from build123d import *

# Parameters (mm, degrees)
F0_W     = 38.1
F0_H     = 38.1
F1_DEPTH = 25.4
F3_DEPTH = 50.8
F4_DEPTH = 6.35


with BuildPart() as f1:
    # F0 (on Front) → F1 (new body)
    with BuildSketch(Plane.XZ):
        with Locations((19.05, 19.05)):
            Rectangle(F0_W, F0_H)
    extrude(amount=F1_DEPTH)

    # F2 (on face) → F3 (cut)
    with BuildSketch(Plane.YZ.offset(38.1)):
        Polygon((-12.6932453566, 11.4907970736), (-12.6932453566, 38.1), (-25.4, 38.1), (-25.4, 11.4952089814), (-25.3932453566, 11.4907970736), align=None)
    extrude(amount=-F3_DEPTH, mode=Mode.SUBTRACT)

    # F4 (cut): a face of the model
    f4_faces = [f1.faces().sort_by_distance(p)[0] for p in [
        (19.05, -6.3466226783, 38.1),
    ]]
    extrude(f4_faces, amount=-F4_DEPTH, mode=Mode.SUBTRACT)


solid = f1.part
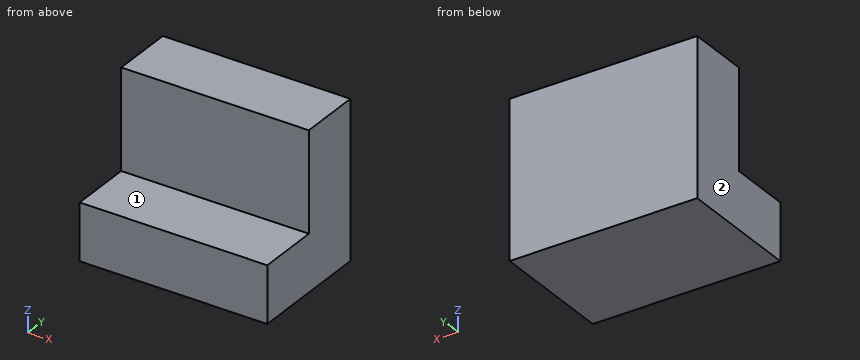
Can you work these out from the model? Positions are in its coordinate system, mm. Face numbers are marked on the shaded views. A direction names the side the tool comes from. Give positions to 0.01 mm unless a question says otherwise; leave off trailing zeros. Loops run counter-clockwise (first coordinate to the right, second up) from the corner with the lowest first, then second, coordinate; pieces in that order, holes last. Notation, with made-up numbers: M 25.25,-37 L 37.25,-37 A15 cw 37.25,-25 Z; hole C 51.25,64.5 d1. An arc over 180 degrees is marked long. One line per item, written item: value. Start each with the question number.
1) If we section it at B-B, the plane z = 12: Write out the boundary of the cut face in (x, y).
2) On a 3-axis mill with a long thin cutter (end or side, diameter ignored), from which of +Z, -Z, +X, -X, +Y, -Y can I reach the whole of each face in a straight line? I mean the marked faces 1 and 2. Say none if no direction works.
3) If I drill on line 1 (Y direction, x = 26, z = 23); line 2 (Z direction, x = 34.5, y = -23), over which ranges is the centre line in solid material (lowest first)? Write a range as [from, to].
4) If we section it at C-C, the plane y = -21.75: Write out the boundary of the cut face in (x, z), and give its area (3 significant figures).
5) I'm going to push a flat-ended pin straight in: pin 1 (2 mm diameter, centred on x = 25, y = -14.5, fed in from +Z). Where does the tip first touch, or does it pass through?
Completed:
1. outline: M 0,-12.69 L 38.1,-12.69 L 38.1,0 L 0,0 Z
2. face 1: +Z, +X, -X, -Y
2. face 2: +Z, -Z, -X, +Y, -Y
3. line 1: y = [-12.69, 0]
3. line 2: z = [0, 11.49]
4. outline: M 0,0 L 38.1,0 L 38.1,11.49 L 0,11.49 Z
4. area: 438 mm^2
5. pin 1: stops at z = 11.49
